Check sheet for the modelled part. Datum: model origin and axes. Units: mm. A direction names the side the tool comes from. Round coordinates to 2 decimals unless told otherwise and drop trailing zeros. Order: outer loops, then holes, each group sorted by start corner. A loop starts at its lowest first (then second) coordinate and runs counter-clockwise, first axis right, second up. Notation, with made-up numbers: (23.25, 3) -> (56.25, 3) arc R31 ccw to (56.25, 30) -> close; hole circle Ø2 at (-4, -15). An arc over 180 degrees is marked (long way). Answer in a Markdown table with one row per item. Add a question column.
1. Sectioned sample at B-B, the plane z = 6.5. Count the separate pieces of the cut face and the enclosed holes in it, then the cut area to 3 significant figures.
2. Material ranges on L1, parallel to Y at x = -37.5, z = 5; L2, parallel to X at y = 10.5, z = 3.25; L3, parallel to Y at x = 36, z = 3.5, recorded low to high. Write a range as from..to.
3. Access from +Z, -Z, +X, -X, +Y, -Y to the whole of each face (thin tool, end or side, straight path). Record for faces 4 (the flat face through (10, -10, 4)), 5 (the cylindrical face through (9.538, -42.954, 8.986)), 6 (the cylindrical face through (26.529, 28.303, 3.944)).
4. Draft check along X on faces 1 (the flat face through (1, 108.253, 5)), 2 (the flat face through (-93.313, 54.884, 4.93)), 3 (the cylindrical face through (7.771, -33.336, 3.944)). Enter one of: +X half, -X half, draft (parallel to the pull), parting line (faces both ways), or undercut.
5. Sectioned sample at C-C, the plane y = 93. Record the boundary of the cut face in (x, z), then the cut area to 3 significant figures.
6. Sectioned sample at D-D, the plane x = -97. Record the boundary of the cut face in (y, z), then the cut area to 3 significant figures.
7. Depth check by flat-ended pin: P1, Ø4, axis at x = 74.5, z = 7.5, coming from the -Y side; P2, Ø9, axis at x = -28.68, y = -24.93, coming from the +Z side; P3, Ø2, axis at y = 68, z = 7.5, coming from the -X side. Enter the tip coordinate at first touch or a pass-through.
8. Sectioned sample at A-A, the plane x = 0. Record the boundary of the cut face in (y, z), then the cut area to 3 significant figures.
```python
from build123d import *

# Parameters (mm, degrees)
F1_DEPTH = 10
F5_D     = 8
F5_DEPTH = 15
F6_D     = 8
F6_DEPTH = 15


with BuildPart() as f1:
    # F0 (on Top) → F1 (new body)
    with BuildSketch(Plane.XY):
        Polygon((62.5, -108.253175), (125, 0), (62.5, 108.253175), (-62.5, 108.253175), (-125, 0), (-62.5, -108.253175), align=None)
    extrude(amount=F1_DEPTH)

    # F2 (on Front) → F3 (revolve, cut)
    with BuildSketch(Plane.XZ):
        Polygon((-23.5, 4), (-23.5, -10), (0, -10), (0, 18), (-44, 18), (-44, 8), (-13, 8), (-13, 4), align=None)
    revolve(axis=Axis((0, 0, -2.490325), (0, 0, -1)), mode=Mode.SUBTRACT)

    # F5
    with Locations(Plane.XY.offset(10)):
        with Locations((-9.826663, 50.5538), (38.867543, 33.78704), (48.694207, -16.76676), (9.826663, -50.5538), (-38.867543, -33.78704), (-48.694207, 16.76676)):
            Hole(F5_D / 2, depth=F5_DEPTH)

    # F6
    with Locations(Plane.XY.offset(10)):
        with Locations((-7.250742, 37.301833), (28.678964, 24.930243), (35.929706, -12.37159), (7.250742, -37.301833), (-28.678964, -24.930243), (-35.929706, 12.37159)):
            Hole(F6_D / 2, depth=F6_DEPTH)


solid = f1.part
```
Answer key:
| question | item | result |
|---|---|---|
| 1 | separate pieces | 1 |
| 1 | enclosed holes | 13 |
| 1 | area | 39,500 mm² |
| 2 | L1 | y = -108.25..-37.55, -30.03..8.69, 16.05..108.25 |
| 2 | L2 | x = -118.94..-39.46, -32.39..-21.02, 21.02..118.94 |
| 2 | L3 | y = -108.25..-16.37, -8.37..31, 36.58..108.25 |
| 3 | face 4 | -Z |
| 3 | face 5 | +Z |
| 3 | face 6 | +Z, -Z |
| 4 | face 1 | draft |
| 4 | face 2 | -X half |
| 4 | face 3 | undercut |
| 5 | outline | (-71.31, 0) -> (71.31, 0) -> (71.31, 10) -> (-71.31, 10) -> close |
| 5 | area | 1,430 mm² |
| 6 | outline | (-48.5, 0) -> (48.5, 0) -> (48.5, 10) -> (-48.5, 10) -> close |
| 6 | area | 970 mm² |
| 7 | P1 | stops at y = -90.93 |
| 7 | P2 | stops at z = 8 |
| 7 | P3 | stops at x = -86.32 |
| 8 | outline | (-108.25, 0) -> (-23.5, 0) -> (-23.5, 4) -> (-13, 4) -> (-13, 8) -> (-44, 8) -> (-44, 10) -> (-108.25, 10) -> close; (13, 4) -> (23.5, 4) -> (23.5, 0) -> (108.25, 0) -> (108.25, 10) -> (44, 10) -> (44, 8) -> (13, 8) -> close |
| 8 | area | 1,700 mm² |
